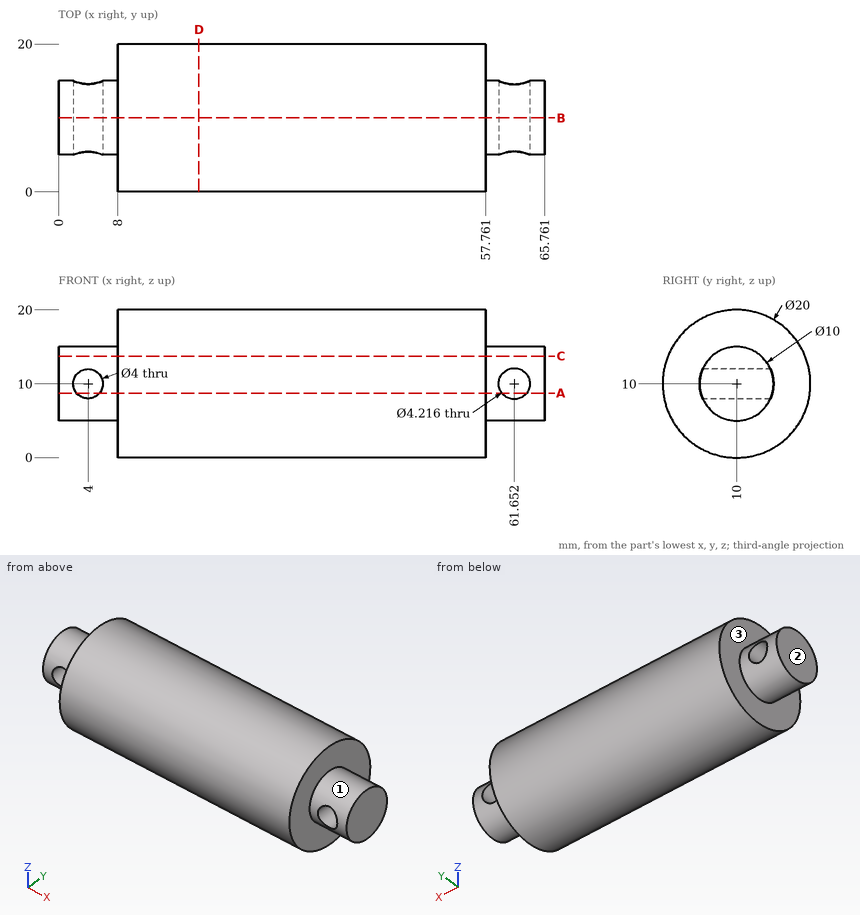
Check sheet for the drawn part. Datum: minimum x, y, z corner. Units: mm. A direction names the side the tool comes from. Give positions to 0.01 mm unless a question says otherwise; leave off trailing zeros. Order: outer loops, then holes, each group sorted by start corner. A loop starts at its lowest first (then second) coordinate and runs counter-clockwise, first axis right, second up. Notation, with made-up numbers: (53.5, 44) - (98.5, 44) arc R16 cw to (98.5, 62) - close; hole circle Ø9 at (75, 1.25). An arc over 180 degrees is marked (long way). Answer as a JSON object with one key per item and string values.
(1) Material ranges on line 1 (X direction, y = 9, z = 10) (1 decimal); line 2 (X direction, y = 8.5, z = 19); line 3 (Y direction, x = 35.5, z = 10), recorded low to high.
Report:
{"line 1": "0 to 2, 6 to 59.5, 63.8 to 65.8", "line 2": "8 to 57.76", "line 3": "0 to 20"}
(2) Cross-section at D-D (x = 19). Record the cut outline in (y, z).
Report:
{"outline": "circle Ø20 at (10, 10)"}
(3) Cross-section at A-A (z = 8.75). State how many separate pieces and enclosed holes the cut face has, then the cut area to 3 significant figures.
Report:
{"separate pieces": "3", "enclosed holes": "0", "area": "1,080 mm^2"}
(4) Tool access check on the marked faces 1, 2 and 3. Record the directions out of +Z, -Z, +X, -X, +Y, -Y that give a thin tool (end or side, any length) a straight path to the whole face; none if there is none.
Report:
{"face 1": "+X", "face 2": "+Z, -Z, -X, +Y, -Y", "face 3": "-X"}
(5) Depth check by flat-ended pin: pin 1 Ø4 at (x, y) = (7.5, 5) entering from +Z; pin 2 Ø3.5 at (x, z) = (4, 10) entering from +Y; pin 3 Ø1 at (y, z) = (15, 5.5) entering from -X; pin 4 Ø6 at (x, y) = (54.5, 2.5) entering from +Z. Enter the tip coordinate at first touch or a pass-through.
Report:
{"pin 1": "z = 19.52", "pin 2": "through", "pin 3": "x = 8", "pin 4": "z = 18.93"}
(6) Cross-section at C-C (z = 13.75). Record the cut outline in (x, y).
Report:
{"outline": "(0, 6.69) - (8, 6.69) - (8, 0.73) - (57.76, 0.73) - (57.76, 6.69) - (65.76, 6.69) - (65.76, 13.31) - (57.76, 13.31) - (57.76, 19.27) - (8, 19.27) - (8, 13.31) - (0, 13.31) - close"}
(7) Cross-section at B-B (y = 10). Record the cut outline in (x, z).
Report:
{"outline": "(0, 5) - (8, 5) - (8, 0) - (57.76, 0) - (57.76, 5) - (65.76, 5) - (65.76, 15) - (57.76, 15) - (57.76, 20) - (8, 20) - (8, 15) - (0, 15) - close; hole circle Ø4 at (4, 10); hole circle Ø4.22 at (61.65, 10)"}
